Check sheet for the modelled part. Datum: model origin and axes. Units: mm. A direction names the side the tool comes from. Round coordinates to 2 decimals unless told otherwise and drop trailing zeros. Write each loop counter-clockwise with the first axis right and the second up, starting at its lowest first coordinate (ties: lowest second). Pieces come first, ordered by that corner, then holes. Notation, with made-up numbers: (-32.5, 31) -> (-28.5, 31) arc R19 ccw to (-28.5, 49) -> close; hole circle Ø10 at (74, 84.5). An arc over 180 degrees is marked (long way). One line per item, written item: value.
from build123d import *

# Parameters (mm, degrees)
SZKIC1_W                    = 4
SZKIC1_H                    = 1
DODANIE_WYCI_GNI_CIE1_DEPTH = 5
SZKIC2_W                    = 4
SZKIC2_H                    = 1
DODANIE_WYCI_GNI_CIE2_DEPTH = 4.5
SZKIC3_W                    = 4
SZKIC3_H                    = 1
DODANIE_WYCI_GNI_CIE3_DEPTH = 1
SZKIC4_W                    = 4
SZKIC4_H                    = 1
DODANIE_WYCI_GNI_CIE4_DEPTH = 1
SZKIC5_W                    = 4
SZKIC5_H                    = 1
DODANIE_WYCI_GNI_CIE5_DEPTH = 3
SZKIC6_W                    = 4
SZKIC6_H                    = 1
DODANIE_WYCI_GNI_CIE6_DEPTH = 2.5
SZKIC8_W                    = 3.5
SZKIC8_H                    = 0.5
DODANIE_WYCI_GNI_CIE7_DEPTH = 3.9
SZKIC9_R                    = 1
WYTNIJ_WYCI_GNI_CIE2_DEPTH  = 3.9
ZAOKR_GLENIE1_R             = 0.25
SZKIC10_W                   = 1
SZKIC10_H                   = 1
WYTNIJ_WYCI_GNI_CIE3_DEPTH  = 1


with BuildPart() as part:
    # Szkic1 → Dodanie-wyciągnięcie1 (new body)
    with BuildSketch(Plane(origin=(0, 0, 0), x_dir=(1, 0, 0), z_dir=(0, 1, 0))):
        Rectangle(SZKIC1_W, SZKIC1_H)
    extrude(amount=DODANIE_WYCI_GNI_CIE1_DEPTH)

    # Szkic2 → Dodanie-wyciągnięcie2 (add)
    with BuildSketch(Plane.XY.offset(0.5)):
        with Locations((0, 4.5)):
            Rectangle(SZKIC2_W, SZKIC2_H)
    extrude(amount=DODANIE_WYCI_GNI_CIE2_DEPTH)

    # Szkic3 → Dodanie-wyciągnięcie3 (add)
    with BuildSketch(Plane(origin=(0, 5, 0), x_dir=(1, 0, 0), z_dir=(0, 1, 0))):
        Rectangle(SZKIC3_W, SZKIC3_H)
    extrude(amount=DODANIE_WYCI_GNI_CIE3_DEPTH)

    # Szkic4 → Dodanie-wyciągnięcie4 (add)
    with BuildSketch(Plane(origin=(0, 0, -0.5), x_dir=(-1, 0, 0), z_dir=(0, 0, -1))):
        with Locations((0, 5.5)):
            Rectangle(SZKIC4_W, SZKIC4_H)
    extrude(amount=DODANIE_WYCI_GNI_CIE4_DEPTH)

    # Szkic5 → Dodanie-wyciągnięcie5 (add)
    with BuildSketch(Plane(origin=(0, 6, 0), x_dir=(1, 0, 0), z_dir=(0, 1, 0))):
        with Locations((0, 1)):
            Rectangle(SZKIC5_W, SZKIC5_H)
    extrude(amount=DODANIE_WYCI_GNI_CIE5_DEPTH)

    # Szkic6 → Dodanie-wyciągnięcie6 (add)
    with BuildSketch(Plane(origin=(0, 5, 0), x_dir=(1, 0, 0), z_dir=(0, 1, 0))):
        with Locations((0, -3.5)):
            Rectangle(SZKIC6_W, SZKIC6_H)
    extrude(amount=DODANIE_WYCI_GNI_CIE6_DEPTH)

    # Szkic8 → Dodanie-wyciągnięcie7 (add)
    with BuildSketch(Plane.XZ):
        Rectangle(SZKIC8_W, SZKIC8_H)
    extrude(amount=DODANIE_WYCI_GNI_CIE7_DEPTH)

    # Szkic9 → Wytnij-wyciągnięcie2 (cut)
    with BuildSketch(Plane.XY.offset(0.25)):
        with Locations((0, -2.4)):
            Circle(SZKIC9_R)
    extrude(amount=-WYTNIJ_WYCI_GNI_CIE2_DEPTH, mode=Mode.SUBTRACT)

    # Zaokrąglenie1
    zaokr_glenie1_edges = [part.edges().sort_by_distance(p)[0] for p in [
        (-1.75, 0, 0),
        (0, 0, -0.25),
        (1.75, 0, 0),
        (0, 0, 0.25),
        (-1.75, -3.9, 0),
        (1.75, -3.9, 0),
    ]]
    fillet(zaokr_glenie1_edges, radius=ZAOKR_GLENIE1_R - 0.0001)  # a hair under: the kernel refuses the full size

    # Szkic10 → Wytnij-wyciągnięcie3 (cut)
    with BuildSketch(Plane.XY.offset(4)):
        with Locations((0, 6.352223481)):
            Rectangle(SZKIC10_W, SZKIC10_H)
    extrude(amount=-WYTNIJ_WYCI_GNI_CIE3_DEPTH, mode=Mode.SUBTRACT)


solid = part.part
Item 1: Sectioned sample at A-A (y = 7.25). Enter the section's corners in (x, z), then the cut area to 3 significant figures.
Result set:
outline: (-2, -1.5) -> (2, -1.5) -> (2, -0.5) -> (-2, -0.5) -> close; (-2, 3) -> (2, 3) -> (2, 4) -> (-2, 4) -> close
area: 8.00 mm^2
Item 2: Sectioned sample at C-C (z = 3.5). Enter the section's corners in (x, y), then the cut area to 3 significant figures.
Result set:
outline: (-2, 4) -> (2, 4) -> (2, 7.5) -> (-2, 7.5) -> close; hole (-0.5, 5.85) -> (0.5, 5.85) -> (0.5, 6.85) -> (-0.5, 6.85) -> close
area: 13.0 mm^2
Item 3: Material ranges on line 1 along Y through (x, z) = (0, 0.1); line 2 along Z through (x, y) = (-1.8, 6.75); line 3 along Z through (x, y) = (1.35, 5.5), recorded low to high.
Result set:
line 1: -3.9 to -3.4, -1.4 to 6
line 2: -1.5 to -0.5, 3 to 4
line 3: -1.5 to 0.5, 3 to 4
Item 4: Sectioned sample at D-D (y = -2.4). Enter the section's corners in (x, z).
Result set:
outline: (-1.75, -0.25) -> (-1, -0.25) -> (-1, 0.25) -> (-1.75, 0.25) -> close; (1, -0.25) -> (1.75, -0.25) -> (1.75, 0.25) -> (1, 0.25) -> close
Item 5: Depth check by flat-ended pin: pin 1 (1.1 mm diameter, centred on x = 0, z = 3.5, fed in from -Y); pin 2 (1.5 mm diameter, centred on x = 0, y = 1.5, fed in from +Z); pin 3 (0.8 mm diameter, centred on x = 0.5, z = 2, fed in from +Y). Enter the tip coordinate at first touch or a pass-through.
Result set:
pin 1: y = 4
pin 2: z = 0.5
pin 3: y = 5
Item 6: Release check for a two-part mould opening along Z. For faces 5 (the flat face through (2, 4.8, 1.3)), 6 (the flat face through (0, 5.5, 0.5)), 7 (the flat face through (0, -1, 0.25)), 8 (the flat face through (0, 7, -1.5)) record: pulls with the +Z half, pulls with the -Z half, needs draft (parallel to the pull), parting line crosses it, or undercut.
Result set:
face 5: needs draft
face 6: undercut
face 7: pulls with the +Z half
face 8: pulls with the -Z half
Item 7: Tool access check on faces 1 (the flat face through (0, 4, 3)), 2 (the flat face through (0, 5.7, 4)), 3 (the flat face through (0.5, 6.3, 3.5)), 4 (the flat face through (0, 7, -0.5)). Record the directions out of +Z, -Z, +X, -X, +Y, -Y that give a thin tool (end or side, any length) a straight path to the whole face; none if there is none.
Result set:
face 1: +Z, +X, -X, -Y
face 2: +Z, +X, -X, +Y
face 3: +Z
face 4: +X, -X, +Y
Item 8: Sectioned sample at B-B (x = 0). State how many separate pieces and enclosed holes the cut face has, then the cut area to 3 significant figures.
Result set:
separate pieces: 3
enclosed holes: 0
area: 17.0 mm^2
